Check sheet for the drawn part. Datum: minimum x, y, z corner. Units: mm. A direction names the side the tool comes from. Coordinates: 2 decimals unless noted, no trailing zeros. Write each loop counter-clockwise with the first axis right and the second up, starting at its lowest first coordinate (ties: lowest second). Pieces come first, ordered by that corner, then holes. Notation, with made-up numbers: (-37.75, 27) -> (8.25, 27) arc R19 cw to (8.25, 53) -> close; hole circle Ø6 at (15, -13.75). An arc over 180 degrees is marked (long way). Answer in a Markdown table with one row per item. Add a question column.
1. Depth check by flat-ended pin: P1, Ø3.5, axis at x = 68, z = 8, coming from the -Y side; P2, Ø4, axis at y = 3.5, z = 18.5, coming from the -X side; P3, Ø2, axis at x = 9, z = 6.5, coming from the -Y side. Enter the tip coordinate at first touch or a pass-through.
2. Cross-section at A-A on z = 7.5. Record the cut outline in (x, y).
3. Scan lines: L1, parallel to X at y = 4, z = 42.5; L2, parallel to Z at x = 20, y = 7.2; L3, parallel to Z at x = 39.5, y = 8.5. Record each from-to range of solid material in increasing order. Write a range as from..to.
4. Cross-section at B-B on x = 67.5. Record the cut outline in (y, z), and give its area (3 significant figures).
5. Cross-section at C-C on y = 5. Give the number of separate pieces and of enclosed holes in the cut face, and give its area (3 significant figures).
6. Set-up check for the marked faces 1 and 2: record each of +Z, -Z, +X, -X, +Y, -Y from which the full face is reachable in a straight line by a thin tool's end or side.
7. Cross-section at D-D on z = 29. Record the cut outline in (x, y).
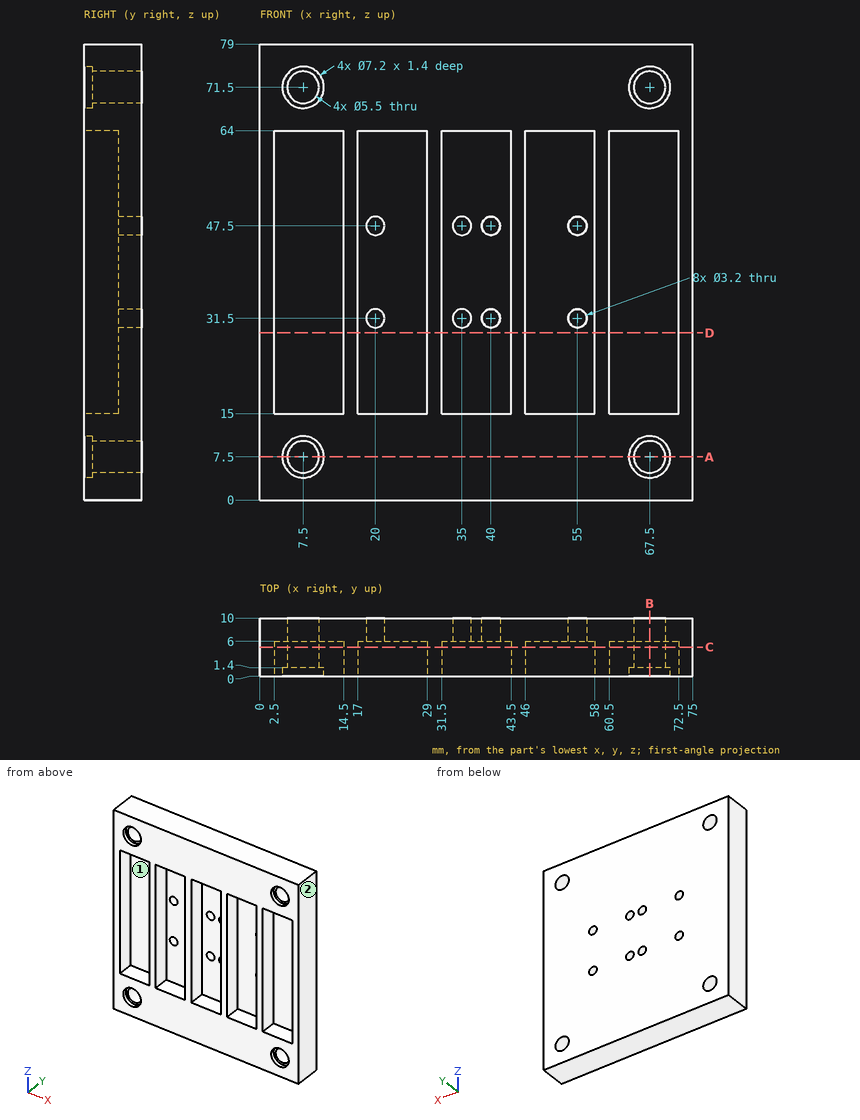
Results found:
| question | item | result |
|---|---|---|
| 1 | P1 | passes through |
| 1 | P2 | stops at x = 0 |
| 1 | P3 | stops at y = 1.4 |
| 2 | outline | (0, 0) -> (3.9, 0) -> (3.9, 1.4) -> (4.75, 1.4) -> (4.75, 10) -> (0, 10) -> close; (10.25, 1.4) -> (11.1, 1.4) -> (11.1, 0) -> (63.9, 0) -> (63.9, 1.4) -> (64.75, 1.4) -> (64.75, 10) -> (10.25, 10) -> close; (70.25, 1.4) -> (71.1, 1.4) -> (71.1, 0) -> (75, 0) -> (75, 10) -> (70.25, 10) -> close |
| 3 | L1 | x = 0..2.5, 14.5..17, 29..31.5, 43.5..46, 58..60.5, 72.5..75 |
| 3 | L2 | z = 0..29.9, 33.1..45.9, 49.1..79 |
| 3 | L3 | z = 0..29.98, 33.02..45.98, 49.02..79 |
| 4 | outline | (0, 0) -> (10, 0) -> (10, 4.75) -> (1.4, 4.75) -> (1.4, 3.9) -> (0, 3.9) -> close; (0, 11.1) -> (1.4, 11.1) -> (1.4, 10.25) -> (10, 10.25) -> (10, 68.75) -> (1.4, 68.75) -> (1.4, 67.9) -> (0, 67.9) -> (0, 64) -> (6, 64) -> (6, 15) -> (0, 15) -> close; (0, 75.1) -> (1.4, 75.1) -> (1.4, 74.25) -> (10, 74.25) -> (10, 79) -> (0, 79) -> close |
| 4 | area | 381 mm^2 |
| 5 | separate pieces | 1 |
| 5 | enclosed holes | 9 |
| 5 | area | 2,890 mm^2 |
| 6 | face 1 | -Y |
| 6 | face 2 | +Z, -Z, +X, +Y, -Y |
| 7 | outline | (0, 0) -> (2.5, 0) -> (2.5, 6) -> (14.5, 6) -> (14.5, 0) -> (17, 0) -> (17, 6) -> (29, 6) -> (29, 0) -> (31.5, 0) -> (31.5, 6) -> (43.5, 6) -> (43.5, 0) -> (46, 0) -> (46, 6) -> (58, 6) -> (58, 0) -> (60.5, 0) -> (60.5, 6) -> (72.5, 6) -> (72.5, 0) -> (75, 0) -> (75, 10) -> (0, 10) -> close |
